```python
from build123d import *

# Parameters (mm, degrees)
SKETCH_1_W               = 20
SKETCH_1_H               = 15
EXTRUDE_1_DEPTH          = 1
SM_START                 = -7.5
SM_EDGE_FLANGE_2_DEPTH   = 15
SM_EDGE_FLANGE_2_2_DEPTH = 15
SM_EDGE_FLANGE_3_DEPTH   = 15
SM_EDGE_FLANGE_3_2_DEPTH = 15
SKETCH_27_R              = 1.5
CUT_EXTRUDE_1_DEPTH      = 5
SKETCH_28_R              = 1.5
CUT_EXTRUDE_2_DEPTH      = 10


# Read off the part's stored shape, not the designer's step: Ребро-кромка2, Ребро-кромка3
with BuildPart() as part:
    # Sketch 1 → Бобышка-Вытянуть1 (new body)
    with BuildSketch(Plane(origin=(0, 0, 0), x_dir=(1, 0, 0), z_dir=(0, 1, 0))):
        Rectangle(SKETCH_1_W, SKETCH_1_H)
    extrude(amount=EXTRUDE_1_DEPTH)

    # Ребро-кромка2 outline → Ребро-кромка2 (cut)
    with BuildSketch(Plane.XY.offset(SM_START)):
        with BuildLine():
            Line((-10, 0), (-9.923154453, 0.15755672))
            ThreePointArc((-9.923154453, 0.15755672), (-9.36984228, 0.772072144), (-8.574963384, 1))
            Line((-8.574963384, 1), (-10, 1))
            Line((-10, 1), (-10, 0))
        make_face()
        with BuildLine():
            Line((10, 1), (8.574963384, 1))
            ThreePointArc((8.574963384, 1), (9.36984228, 0.772072144), (9.923154453, 0.15755672))
            Line((9.923154453, 0.15755672), (10, 0))
            Line((10, 0), (10, 1))
        make_face()
    extrude(amount=SM_EDGE_FLANGE_2_DEPTH, mode=Mode.SUBTRACT)

    # Sm Edge Flange 2 2 outline → Sm Edge Flange 2 2 (add)
    with BuildSketch(Plane.XY.offset(SM_START)):
        with BuildLine():
            Line((-8.574963384, 0), (-10, 0))
            Line((-10, 0), (-45.458701448, -72.701111797))
            Line((-45.458701448, -72.701111797), (-44.559907402, -73.139482943))
            Line((-44.559907402, -73.139482943), (-9.024360407, -0.280814427))
            ThreePointArc((-9.024360407, -0.280814427), (-8.839923016, -0.075975952), (-8.574963384, 0))
        make_face()
        with BuildLine():
            Line((10, 0), (8.574963384, 0))
            ThreePointArc((8.574963384, 0), (8.839923016, -0.075975952), (9.024360407, -0.280814427))
            Line((9.024360407, -0.280814427), (44.559907402, -73.139482943))
            Line((44.559907402, -73.139482943), (45.458701448, -72.701111797))
            Line((45.458701448, -72.701111797), (10, 0))
        make_face()
    extrude(amount=SM_EDGE_FLANGE_2_2_DEPTH)

    # Ребро-кромка3 outline → Ребро-кромка3 (cut)
    with BuildSketch(Plane.XY.offset(SM_START)):
        with BuildLine():
            ThreePointArc((-43.935212466, -71.858668517), (-44.488524639, -72.473183941), (-45.283403536, -72.701111797))
            Line((-45.283403536, -72.701111797), (-45.458701448, -72.701111797))
            Line((-45.458701448, -72.701111797), (-44.559907402, -73.139482943))
            Line((-44.559907402, -73.139482943), (-43.935212466, -71.858668517))
        make_face()
        with BuildLine():
            Line((44.559907402, -73.139482943), (45.458701448, -72.701111797))
            Line((45.458701448, -72.701111797), (45.283403536, -72.701111797))
            ThreePointArc((45.283403536, -72.701111797), (44.488524639, -72.473183941), (43.935212466, -71.858668517))
            Line((43.935212466, -71.858668517), (44.559907402, -73.139482943))
        make_face()
    extrude(amount=SM_EDGE_FLANGE_3_DEPTH, mode=Mode.SUBTRACT)

    # Sm Edge Flange 3 2 outline → Sm Edge Flange 3 2 (add)
    with BuildSketch(Plane.XY.offset(SM_START)):
        with BuildLine():
            Line((-55.346099508, -72.701111797), (-45.458701448, -72.701111797))
            Line((-45.458701448, -72.701111797), (-44.834006512, -71.42029737))
            ThreePointArc((-44.834006512, -71.42029737), (-45.018443903, -71.625135845), (-45.283403536, -71.701111797))
            Line((-45.283403536, -71.701111797), (-55.346099508, -71.701111797))
            Line((-55.346099508, -71.701111797), (-55.346099508, -72.701111797))
        make_face()
        with BuildLine():
            Line((45.458701448, -72.701111797), (55.346099508, -72.701111797))
            Line((55.346099508, -72.701111797), (55.346099508, -71.701111797))
            Line((55.346099508, -71.701111797), (45.283403536, -71.701111797))
            ThreePointArc((45.283403536, -71.701111797), (45.018443903, -71.625135845), (44.834006512, -71.42029737))
            Line((44.834006512, -71.42029737), (45.458701448, -72.701111797))
        make_face()
    extrude(amount=SM_EDGE_FLANGE_3_2_DEPTH)

    # Эскиз27 → Вырез-Вытянуть1 (cut)
    with BuildSketch(Plane(origin=(0, -71.701111797, 0), x_dir=(1, 0, 0), z_dir=(0, 1, 0))):
        with Locations(Location((-48.996099508, 0, 0), (0, 0, 270))):
            Circle(SKETCH_27_R)
        with Locations(Location((48.996099508, 0, 0), (0, 0, 270))):
            Circle(SKETCH_27_R)
    extrude(amount=-CUT_EXTRUDE_1_DEPTH, mode=Mode.SUBTRACT)

    # Эскиз28 → Вырез-Вытянуть2 (cut)
    with BuildSketch(Plane(origin=(0, 1, 0), x_dir=(1, 0, 0), z_dir=(0, 1, 0))):
        with Locations(Location((-5.804963384, 0, 0), (0, 0, 270))):
            Circle(SKETCH_28_R)
    extrude(amount=-CUT_EXTRUDE_2_DEPTH, mode=Mode.SUBTRACT)


solid = part.part
```
CAD build for the part. Positions are in the model's coordinates, mm. A direction names the side the tool comes from. Give positions to 0.01 mm unless a question says otherwise; leave off trailing zeros. Order: outer loops, then holes, each group sorted by start corner. A loop starts at its lowest first (then second) coordinate and runs counter-clockwise, first axis right, second up. Notation, with made-up numbers: M -14.75,-7.75 L -2.75,-7.75 A19 cw -2.75,27.25 Z; hole C 11.25,-39 d1. An arc over 180 degrees is marked long. Put each result on its own line as item: value. Start each with the question number.
(1) Drill centre lines: line 1 along X through (y, z) = (-72.3, 0); line 2 along X through (y, z) = (-72.25, 0); line 3 along Y through (x, z) = (1, 7). Where is each one in solid material? Low to high.
(2) Saw through at A-A, the plane y = -49.5. Write the cut outline in (x, z).
(3) Which spindle directions (+Z, -Z, +X, -X, +Y, -Y) get a long thin tool onto all of the face, cutting with end or side? Do faces 1 (the flat face through (-26.724, -36.571, -0.105)), 2 (the flat face through (52, -71.701, 0)), 3 (the flat face through (-51, -71.701, 0)). Say none if no direction does.
(4) Flat gauge pins, fed straight in: pin 1 Ø1.8 at (x, z) = (49, 0) entering from +Y; pin 2 Ø1.5 at (y, z) = (-17.5, -3) entering from -X; pin 3 Ø5 at (y, z) = (-25.5, 2.5) entering from -X; pin 4 Ø3 at (y, z) = (-23.5, -3) entering from -X. Where does each tip first touch, or does it go through?
(5) Saw through at B-B, the plane z = 0. Give the number of separate pieces and of enclosed holes in the cut face, then the cut area to 3 significant figures.
(6) Mould opens along X. For faces 4 (the flat face through (52, -72.701, 0)), 5 (the flat face through (26.235, -35.569, -0.105)) say: +X half, -X half, draft (parallel to the pull), parting line (faces both ways), or undercut.
(7) Saw through at C-C, the plane z = -5. Write the cut outline in (x, y).
(8) Saw through at D-D, the plane x = 4. Write the cut outline in (y, z).
Check result:
1. line 1: x = -55.35 to -50.5, -47.5 to -44.26, 44.26 to 47.5, 50.5 to 55.35
1. line 2: x = -55.35 to -50.5, -47.5 to -44.21, 44.21 to 47.5, 50.5 to 55.35
1. line 3: y = 0 to 1
2. outline: M -34.14,-7.5 L -33.03,-7.5 L -33.03,7.5 L -34.14,7.5 Z; M 33.03,-7.5 L 34.14,-7.5 L 34.14,7.5 L 33.03,7.5 Z
3. face 1: +Z, -Z, -Y
3. face 2: +Z, -Z, +X, +Y
3. face 3: +Z, -Z, -X, +Y
4. pin 1: passes through
4. pin 2: stops at x = -18.9
4. pin 3: stops at x = -23.66
4. pin 4: stops at x = -22.19
5. separate pieces: 4
5. enclosed holes: 0
5. area: 192 mm2
6. face 4: draft
6. face 5: undercut
7. outline: M -55.35,-72.7 L -45.28,-72.7 A1.5 ccw -43.94,-71.86 L -9.02,-0.28 A0.5 cw -8.57,0 L 8.57,0 A0.5 cw 9.02,-0.28 L 43.94,-71.86 A1.5 ccw 45.28,-72.7 L 55.35,-72.7 L 55.35,-71.7 L 45.28,-71.7 A0.5 cw 44.83,-71.42 L 9.92,0.16 A1.5 ccw 8.57,1 L -8.57,1 A1.5 ccw -9.92,0.16 L -44.83,-71.42 A0.5 cw -45.28,-71.7 L -55.35,-71.7 Z
8. outline: M 0,-7.5 L 1,-7.5 L 1,7.5 L 0,7.5 Z
